Geometry: final body of the model. Coordinates: model frame, mm. Give positions to 0.01 mm unless a question says otherwise; leave off trailing zeros. Write each loop counter-clockwise with the first axis right and the second up, starting at its lowest first coordinate (ties: lowest second). Pieces come first, ordered by that corner, then holes.
Q1. Section D-D (z = 13). Return the cut outline in (x, y) (3 decimals), plus the area to 3 significant figures.
Q2. Line query: line 1 (Z direction, x = 26.45, y = -2.3); line 2 (X direction, y = -1, z = 25); line 3 (Y direction, x = 15, z = 8.5). Output: solid intervals per line, ascending.
Q3. Pin query (flat end, axial travel): pin 1 Ø5 at (x, z) = (4.85, 59.65) entering from -Y; pin 2 Ø1.1 at (y, z) = (7.5, 20.5) entering from +X; pin 3 Ø1.6 at (x, y) = (23, 6.5) entering from +Z; pin 4 Ø2.5 at (x, z) = (26.45, 59.65) entering from -Y. Return the tip coordinate at first contact, or that it passes through.
Q4. Section B-B (x = 26.45). Return the cut outline in (y, z), plus the area to 3 significant figures.
Q5. Section C-C (x = 4.85). Return the cut outline in (y, z), plus the area to 3 significant figures.
Q6. Section A-A (z = 36). Return the cut outline in (x, y) (3 decimals), plus the area to 3 significant figures.
from build123d import *

# Parameters (mm, degrees)
F1_DEPTH  = 64
F3_DEPTH  = 2
F5_DEPTH  = 2
F7_DEPTH  = 2
F9_DEPTH  = 2
F10_SIZE  = 1
F11_R     = 1.6
F12_DEPTH = 3.001
F13_W     = 11
F13_H     = 5
F14_DEPTH = 1.5
F16_DEPTH = 5
F17_R     = 1.072280415
F18_DEPTH = 1
F20_DEPTH = 3


with BuildPart() as f1:
    # F0 (on Top) → F1 (new body)
    with BuildSketch(Plane.XY):
        with BuildLine():
            Line((28.3, 8), (15.65, 8))
            Line((15.65, 8), (3, 8))
            ThreePointArc((3, 8), (-0.5355339059, 6.5355339059), (-2, 3))
            Line((-2, 3), (-2, -3))
            Line((-2, -3), (15.65, -3))
            Line((15.65, -3), (33.3, -3))
            Line((33.3, -3), (33.3, 3))
            ThreePointArc((33.3, 3), (31.8355339059, 6.5355339059), (28.3, 8))
        make_face()
        Polygon((15.65, 0), (0, 0), (0, 2.2), (0.875, 2.2), (1.75, 3.075), (1.75, 6), (15.65, 6), (29.55, 6), (29.55, 3.075), (30.425, 2.2), (31.3, 2.2), (31.3, 0), align=None, mode=Mode.SUBTRACT)
    extrude(amount=F1_DEPTH)

    # F2 (on face) → F3 (join)
    with BuildSketch(Plane(origin=(0, 0, 0), x_dir=(1, 0, 0), z_dir=(0, 0, -1))):
        with BuildLine():
            ThreePointArc((-2, -3), (-0.5355339059, -6.5355339059), (3, -8))
            Line((3, -8), (28.3, -8))
            ThreePointArc((28.3, -8), (31.8355339059, -6.5355339059), (33.3, -3))
            Line((33.3, -3), (33.3, 3))
            Line((33.3, 3), (-2, 3))
            Line((-2, 3), (-2, -3))
        make_face()
    extrude(amount=F3_DEPTH)

    # F4 (on face) → F5 (cut, through all)
    with BuildSketch(Plane(origin=(0, 8, 0), x_dir=(-1, 0, 0), z_dir=(0, 1, 0))):
        with BuildLine():
            Line((-7.4, 59.5), (-7.4, 64))
            Line((-7.4, 64), (-15.65, 64))
            Line((-15.65, 64), (-23.9, 64))
            Line((-23.9, 64), (-23.9, 59.5))
            ThreePointArc((-23.9, 59.5), (-23.7535533906, 59.1464466094), (-23.4, 59))
            Line((-23.4, 59), (-15.65, 59))
            Line((-15.65, 59), (-7.9, 59))
            ThreePointArc((-7.9, 59), (-7.5464466094, 59.1464466094), (-7.4, 59.5))
        make_face()
    extrude(amount=-F5_DEPTH, mode=Mode.SUBTRACT)

    # F6 (on face) → F7 (cut, through all)
    with BuildSketch(Plane(origin=(0, 8, 0), x_dir=(-1, 0, 0), z_dir=(0, 1, 0))):
        with BuildLine():
            Line((-7.85, 64.5738318563), (-7.85, 59.65))
            ThreePointArc((-7.85, 59.65), (-4.85, 56.65), (-1.85, 59.65))
            Line((-1.85, 59.65), (-1.85, 64.5738318563))
            Line((-1.85, 64.5738318563), (-7.85, 64.5738318563))
        make_face()
        with BuildLine():
            ThreePointArc((-29.45, 59.65), (-26.45, 56.65), (-23.45, 59.65))
            Line((-23.45, 59.65), (-23.45, 64.5738318563))
            Line((-23.45, 64.5738318563), (-29.45, 64.5738318563))
            Line((-29.45, 64.5738318563), (-29.45, 59.65))
        make_face()
    extrude(amount=-F7_DEPTH, mode=Mode.SUBTRACT)

    # F8 (on face) → F9 (cut)
    with BuildSketch(Plane(origin=(0, 0, 0), x_dir=(-1, 0, 0), z_dir=(0, 1, 0))):
        with BuildLine():
            Line((-7.4, 59.5), (-7.4, 64))
            Line((-7.4, 64), (-15.65, 64))
            Line((-15.65, 64), (-23.9, 64))
            Line((-23.9, 64), (-23.9, 59.5))
            ThreePointArc((-23.9, 59.5), (-23.7535533906, 59.1464466094), (-23.4, 59))
            Line((-23.4, 59), (-15.65, 59))
            Line((-15.65, 59), (-7.9, 59))
            ThreePointArc((-7.9, 59), (-7.5464466094, 59.1464466094), (-7.4, 59.5))
        make_face()
    extrude(amount=-F9_DEPTH, mode=Mode.SUBTRACT)

    # F10
    f10_edges = [f1.edges().sort_by_distance(p)[0] for p in [
        (3.7, 0, 64),
        (27.6, 0, 64),
        (0, 1.1, 64),
        (0.4375, 2.2, 64),
        (31.3, 1.1, 64),
        (30.8625, 2.2, 64),
    ]]
    chamfer(f10_edges, length=F10_SIZE)

    # F11 (on face) → F12 (cut, through all)
    with BuildSketch(Plane(origin=(0, 0, 0), x_dir=(-1, 0, 0), z_dir=(0, 1, 0))):
        with Locations((-4.85, 59.65)):
            Circle(F11_R)
        with Locations((-26.45, 59.65)):
            Circle(F11_R)
    extrude(amount=-F12_DEPTH, mode=Mode.SUBTRACT)

    # F13 (on face) → F14 (cut)
    with BuildSketch(Plane.XZ.offset(-6)):
        with Locations((24.05, 41.5)):
            Rectangle(F13_W, F13_H)
    extrude(amount=-F14_DEPTH, mode=Mode.SUBTRACT)

    # F15 (on face) → F16 (join, through all)
    with BuildSketch(Plane.XY.offset(39)):
        with BuildLine():
            Line((29.55, 7.5), (28.3, 7.5))
            ThreePointArc((28.3, 7.5), (28.9312414261, 7.4555060613), (29.55, 7.3229041164))
            Line((29.55, 7.3229041164), (29.55, 7.5))
        make_face()
    extrude(amount=F16_DEPTH)

    # F17 (on face) → F18 (cut)
    with BuildSketch(Plane(origin=(0, 8, 0), x_dir=(-1, 0, 0), z_dir=(0, 1, 0))):
        Polygon((-15.0674888864, 32.9711548984), (-21.5556509793, 29.2659867555), (-20.8310857415, 28.0473995954), (-15.0839583948, 31.324416399), (-7.55834952, 26.9770175219), (-7.55834952, 18.298689276), (-15.0839583948, 13.9512922615), (-22.6260330528, 18.3151569217), (-22.6260330528, 23.7329360098), (-24.0422300994, 23.7329360098), (-24.0422300994, 17.4588505179), (-15.0839565322, 12.3374853283), (-6.1586168595, 17.5247211009), (-6.1586168595, 27.8168544173), align=None)
        with Locations((-23.2353284955, 26.7135389149)):
            Circle(F17_R)
        Polygon((-12.0868515223, 19.9723746628), (-12.0868515223, 25.3138449043), (-13.3068170398, 25.3028552979), (-13.3068170398, 22.0715943724), (-14.3948951736, 25.3028552979), (-15.8236827701, 25.3028552979), (-16.9117599726, 22.060604766), (-16.9117599726, 25.3028552979), (-18.1207358837, 25.3028552979), (-18.1207358837, 19.9723746628), (-16.4281707257, 19.9723746628), (-15.1202799752, 23.9180289209), (-13.7684261426, 19.9723746628), align=None)
    extrude(amount=-F18_DEPTH, mode=Mode.SUBTRACT)

    # F19 (on face) → F20 (cut, through all)
    with BuildSketch(Plane.XZ.offset(3)):
        with BuildLine():
            Line((28.3, 27.75), (22.8, 27.75))
            ThreePointArc((22.8, 27.75), (22.4464466094, 27.6035533906), (22.3, 27.25))
            Line((22.3, 27.25), (22.3, 24.75))
            ThreePointArc((22.3, 24.75), (22.4464466094, 24.3964466094), (22.8, 24.25))
            Line((22.8, 24.25), (28.3, 24.25))
            ThreePointArc((28.3, 24.25), (28.6535533906, 24.3964466094), (28.8, 24.75))
            Line((28.8, 24.75), (28.8, 27.25))
            ThreePointArc((28.8, 27.25), (28.6535533906, 27.6035533906), (28.3, 27.75))
        make_face()
    extrude(amount=-F20_DEPTH, mode=Mode.SUBTRACT)


solid = f1.part
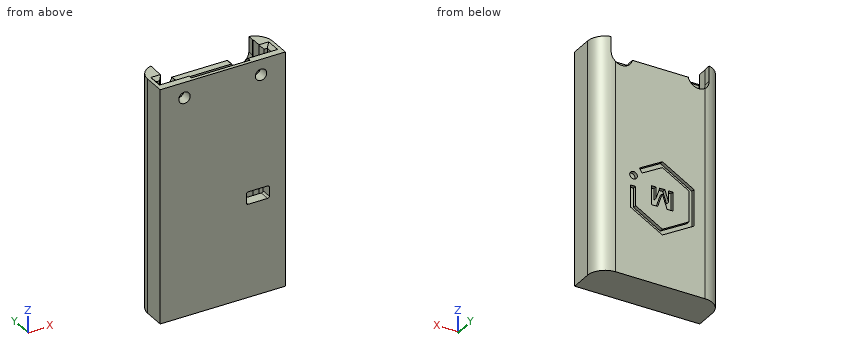
Computed:
1. outline: (-2, -3) - (33.3, -3) - (33.3, 3) arc R5 ccw to (28.3, 8) - (16.243, 8) - (16.243, 7) - (13.944, 7) - (13.944, 8) - (3, 8) arc R5 ccw to (-2, 3) - close; hole (0, 0) - (31.3, 0) - (31.3, 2.2) - (30.425, 2.2) - (29.55, 3.075) - (29.55, 6) - (1.75, 6) - (1.75, 3.075) - (0.875, 2.2) - (0, 2.2) - close
1. area: 200 mm2
2. line 1: z = -2 to 24.25, 27.75 to 58.05, 61.25 to 64
2. line 2: x = -2 to 22.3, 28.8 to 33.3
2. line 3: y = -3 to 0, 6 to 8
3. pin 1: stops at y = -3
3. pin 2: stops at x = 31.37
3. pin 3: stops at z = 59.01
3. pin 4: passes through
4. outline: (-3, -2) - (8, -2) - (8, 56.65) - (6, 56.65) - (6, 44) - (7.5, 44) - (7.5, 39) - (6, 39) - (6, 0) - (0, 0) - (0, 24.25) - (-3, 24.25) - close; (-3, 27.75) - (0, 27.75) - (0, 58.05) - (-3, 58.05) - close; (-3, 61.25) - (0, 61.25) - (0, 63) - (-1, 64) - (-3, 64) - close
4. area: 299 mm2
5. outline: (-3, -2) - (8, -2) - (8, 56.65) - (6, 56.65) - (6, 0) - (0, 0) - (0, 58.05) - (-3, 58.05) - close; (-3, 61.25) - (0, 61.25) - (0, 63) - (-1, 64) - (-3, 64) - close
5. area: 317 mm2
6. outline: (-2, -3) - (33.3, -3) - (33.3, 3) arc R5 ccw to (28.3, 8) - (3, 8) arc R5 ccw to (-2, 3) - close; hole (0, 0) - (31.3, 0) - (31.3, 2.2) - (30.425, 2.2) - (29.55, 3.075) - (29.55, 6) - (1.75, 6) - (1.75, 3.075) - (0.875, 2.2) - (0, 2.2) - close
6. area: 202 mm2
